Check sheet for the modelled part. Datum: model origin and axes. Units: mm. A direction names the side the tool comes from. Coordinates: 2 decimals unless noted, no trailing zeros. Loops run counter-clockwise (first coordinate to the right, second up) from the corner with the lowest first, then second, coordinate; pieces in that order, holes last.
Autodesk Inventor part; units mm, degrees
ref_plane "body_dummy_XY" through (0, 0, 0) normal (0, 0, -1) x (1, 0, 0)
ref_plane "body_dummy_YZ" through (0, 0, 0) normal (1, 0, 0) x (0, -1, 0)
ref_plane "body_dummy_ZX" through (0, 0, 0) normal (0, -1, 0) x (0, 0, -1)
sketch "Sketch_1" plane through (0, 0, 0) normal (0, 0, 1) x (1, 0, 0)
  line L0 (-10, 10) -> (-10, -9)
  line L1 (-10, -9) -> (-9, -10)
  line L2 (-9, -10) -> (9, -10)
  line L3 (9, -10) -> (10, -9)
  line L4 (10, -9) -> (10, 10)
  line L5 (10, 10) -> (-10, 10)
extrude "Extrusion1" add sketch "Sketch_1" along normal mid plane 40
sketch "Sketch_2" plane through (0, 0, 0) normal (0, 1, 0) x (-1, 0, 0)
  line L0 (15, 25) -> (-15, 25)
  line L1 (-15, 25) -> (-15, -25)
  line L2 (-15, -25) -> (15, -25)
  line L3 (15, -25) -> (15, 25)
  line L4 (10, -19) -> (10, 19)
  line L5 (10, 19) -> (9, 20)
  line L6 (9, 20) -> (-9, 20)
  line L7 (-9, 20) -> (-10, 19)
  line L8 (-10, 19) -> (-10, -19)
  line L9 (-10, -19) -> (-9, -20)
  line L10 (-9, -20) -> (9, -20)
  line L11 (9, -20) -> (10, -19)
extrude "Extrusion2" cut sketch "Sketch_2" along normal mid plane 40
sketch "Sketch_3" plane through (0, 0, 0) normal (1, 0, 0) x (0, 1, 0)
  line L0 (15, 25) -> (-15, 25)
  line L1 (-15, 25) -> (-15, -25)
  line L2 (-15, -25) -> (15, -25)
  line L3 (15, -25) -> (15, -20)
  line L4 (15, -20) -> (-9, -20)
  line L5 (-9, -20) -> (-10, -19)
  line L6 (-10, -19) -> (-10, 19)
  line L7 (-10, 19) -> (-9, 20)
  line L8 (-9, 20) -> (15, 20)
  line L9 (15, 20) -> (15, 25)
extrude "Extrusion3" cut sketch "Sketch_3" along normal mid plane 20
sketch "Sketch_4" plane through (0, 0, 0) normal (0, 0, 1) x (1, 0, 0)
  line L0 (0, 59) -> (0, 8)
  line L1 (0, 8) -> (-20, 8)
  line L2 (-20, 8) -> (-20, 20)
  line L3 (-20, 20) -> (-18, 20)
  line L4 (-18, 20) -> (-18, 21.5)
  line L5 (-18, 21.5) -> (-20, 21.5)
  line L6 (-20, 21.5) -> (-20, 24.5)
  line L7 (-20, 24.5) -> (-19, 25.5)
  line L8 (-19, 25.5) -> (-15, 25.5)
  line L9 (-15, 25.5) -> (-15, 35)
  line L10 (-15, 35) -> (-14, 35)
  line L11 (-14, 35) -> (-14, 36)
  line L12 (-14, 36) -> (-12, 36)
  line L13 (-12, 36) -> (-12, 37.09)
  line L14 (-12, 37.09) -> (-14, 37.09)
  line L15 (-14, 37.09) -> (-14, 58)
  line L16 (-14, 58) -> (-13, 59)
  line L17 (-13, 59) -> (0, 59)
  line L18 (0, 59) -> (0, 8)
revolve "Revolution1" add sketch "Sketch_4" angle 360 about axis through (0, 59, 0) along (0, 1, 0)
thread "Thread1"
sketch "Sketch_5" plane through (0, 0, 0) normal (1, 0, 0) x (0, 1, 0)
  line L0 (0, 20) -> (0, 5.0961)
  line L1 (0, 5.0961) -> (-5.7225, 8.4)
  line L2 (-5.7225, 8.4) -> (-5.7225, 19.144)
  line L3 (-5.7225, 19.144) -> (-6.5785, 20)
  line L4 (-6.5785, 20) -> (0, 20)
  line L5 (0, 20) -> (0, 5.0961)
revolve "Revolution2" cut sketch "Sketch_5" angle 360 about axis through (0, 0, 20) along (0, 0, 1)
thread "Thread2"
sketch "Sketch_6" plane through (0, 0, 0) normal (1, 0, 0) x (0, 1, 0)
  line L0 (0, -5.0961) -> (0, -20)
  line L1 (0, -20) -> (-6.5785, -20)
  line L2 (-6.5785, -20) -> (-5.7225, -19.144)
  line L3 (-5.7225, -19.144) -> (-5.7225, -8.4)
  line L4 (-5.7225, -8.4) -> (0, -5.0961)
  line L5 (0, -5.0961) -> (0, -20)
revolve "Revolution3" cut sketch "Sketch_6" angle 360 about axis through (0, 0, -5.0961) along (0, 0, 1)
thread "Thread3"
sketch "Sketch_10" plane through (0, 59, 0) normal (0, 1, 0) x (1, 0, 0)
  line L0 (-3, -0.5) -> (-1, -0.5)
  arc A0 (-0.5, -1) -> (-1, -0.5) centre (-1, -1) ccw
  line L1 (-0.5, -1) -> (-0.5, -3)
  line L2 (-0.5, -3) -> (0.5, -3)
  line L3 (0.5, -3) -> (0.5, -1)
  arc A1 (1, -0.5) -> (0.5, -1) centre (1, -1) ccw
  line L4 (1, -0.5) -> (3, -0.5)
  line L5 (3, -0.5) -> (3, 0.5)
  line L6 (3, 0.5) -> (1, 0.5)
  arc A2 (0.5, 1) -> (1, 0.5) centre (1, 1) ccw
  line L7 (0.5, 1) -> (0.5, 3)
  line L8 (0.5, 3) -> (-0.5, 3)
  line L9 (-0.5, 3) -> (-0.5, 1)
  arc A3 (-1, 0.5) -> (-0.5, 1) centre (-1, 1) ccw
  line L10 (-1, 0.5) -> (-3, 0.5)
  line L11 (-3, 0.5) -> (-3, -0.5)
extrude "Extrusion4" cut sketch "Sketch_10" against normal blind 0.2
sketch "Sketch_11" plane through (0, 59, 0) normal (0, 1, 0) x (1, 0, 0)
  circle A0 centre (0, 0) radius 4.1
  circle A1 centre (0, 0) radius 4
extrude "Extrusion5" cut sketch "Sketch_11" against normal blind 1
ref_plane "body_dummy_XY" through (0, 0, 0) normal (0, 0, -1) x (1, 0, 0)
ref_plane "body_dummy_YZ" through (0, 0, 0) normal (1, 0, 0) x (0, -1, 0)
ref_plane "body_dummy_ZX" through (0, 0, 0) normal (0, -1, 0) x (0, 0, -1)
ref_plane "body_nut_XY" through (0, 27.1, 0) normal (0, 1, 0) x (1, 0, 0)
ref_plane "body_nut_YZ" through (0, 27.1, 0) normal (1, 0, 0) x (0, 0, -1)
ref_plane "body_nut_ZX" through (0, 27.1, 0) normal (0, 0, -1) x (0, 1, 0)
properties part number "AP100-02_BODY"
(1) Draft check along Y on faces 5 (the face through (3.1, 59, 3.1)), 6 (the face through (18, 20, 3)), 7 (the face through (-12.932, 35.507, -5.362)). Enter one of: pulls with the +Y half, pulls with the -Y half, needs draft (parallel to the pull), parting line crosses it, or undercut.
(2) Scan lines: line 1 along X through (y, z) = (0, 15); line 2 along Y through (x, z) = (-14, -3.5); line 3 along Y through (x, z) = (2.5, -9). Record each from-to range of solid material in increasing order.
(3) Gauge pin test, flat ends, axial feed: P1, Ø2, axis at y = 16.5, z = -11, coming from the +X side; P2, Ø15, axis at x = 0, y = 0, coming from the -Z side; P3, Ø0.8, axis at x = -7.5, z = 18.5, coming from the +Y side; P4, Ø1.3, axis at x = -3, z = -19, coming from the +Y side. Record the tip position at first contact, or that the pin passes through.
(4) Set-up check for faces 1 (the face through (1.719, -5.458, -13.697)), 2 (the face through (-8, 10, 19)), 3 (the face through (-12.932, 47.691, -5.362)), 4 (the face through (2.343, 20.76, 17.847)): record each of +Z, -Z, +X, -X, +Y, -Y from which the full face is reachable in a straight line by a thin tool's end or side.
(5) Section check A-A, the plane y = 26.5. Enter the section's corners in (x, z), plus the area to 3 significant figures.
Determined:
1. face 5: pulls with the +Y half
1. face 6: undercut
1. face 7: needs draft
2. line 1: x = -10 to -5.72, 5.72 to 10
2. line 2: y = 8 to 35
2. line 3: y = -10 to -5.15, 5.15 to 59
3. P1: stops at x = 17.32
3. P2: stops at z = -20
3. P3: stops at y = 24.94
3. P4: stops at y = 25.5
4. face 1: -Z
4. face 2: +Z, -X, +Y
4. face 3: +Y
4. face 4: none
5. outline: circle Ø30 at (0, 0)
5. area: 707 mm2
